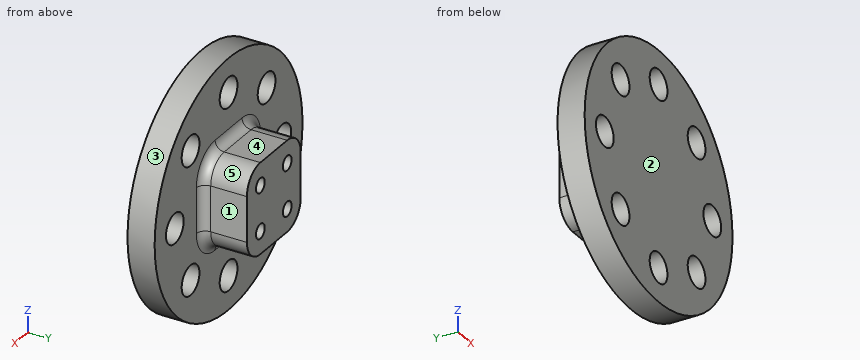
Autodesk Inventor part; units mm, degrees
ref_plane "YZ Plane" through (0, 0, 0) normal (1, 0, 0) x (0, 1, 0)
ref_plane "XZ Plane" through (0, 0, 0) normal (0, 1, 0) x (-1, 0, 0)
ref_plane "XY Plane" through (0, 0, 0) normal (0, 0, 1) x (1, 0, 0)
sketch "Sketch1" plane through (0, 0, 0) normal (0, 1, 0) x (-1, 0, 0)
  circle A0 centre (0, 0) radius 27.5
  dimension "d0" = 55
extrude "Extrusion1" add sketch "Sketch1" along normal blind 6
sketch "Sketch2" plane through (0, 6, 0) normal (0, 1, 0) x (1, 0, 0)
  circle A0 centre (0, 0) radius 27.5
  point P0 (20, 0)
  point P1 (14.1421, 14.1421)
  point P2 (0, 20)
  point P3 (-14.1421, 14.1421)
  point P4 (-20, 0)
  point P5 (-14.1421, -14.1421)
  point P6 (0, -20)
  point P7 (14.1421, -14.1421)
  dimension "d3" = 20
  dimension "d6" = 360
hole "Hole1" at (20, 6, 0) at (14.1421, 6, -14.1421) at (0, 6, -20) at (-14.1421, 6, -14.1421) at (-20, 6, 0) at (-14.1421, 6, 14.1421) at (0, 6, 20) at (14.1421, 6, 14.1421) direction (0, -1, 0) diameter 6.6 depth 8 tip angle 118
sketch "Sketch3" plane through (0, 6, 0) normal (0, 1, 0) x (1, 0, 0)
  circle A0 centre (0, 0) radius 27.5
  line L0 (-5, 10) -> (5, 10)
  line L1 (10, 5) -> (10, -5)
  line L2 (5, -10) -> (-5, -10)
  line L3 (-10, -5) -> (-10, 5)
  arc A1 (-5, 10) -> (-10, 5) centre (-5, 5) ccw
  arc A2 (10, 5) -> (5, 10) centre (5, 5) ccw
  arc A3 (5, -10) -> (10, -5) centre (5, -5) ccw
  arc A4 (-10, -5) -> (-5, -10) centre (-5, -5) ccw
  point P0 (0, 10)
  point P1 (10, 0)
  dimension "d15" = 5
  dimension "d16" = 20
  dimension "d17" = 20
extrude "Extrusion2" add sketch "Sketch3" along normal blind 10 contours L0 A2 L1 A3 L2 A4 L3 A1
sketch "Sketch4" plane through (0, 16, 0) normal (0, 1, 0) x (1, 0, 0)
  arc A0 (-5, 10) -> (-10, 5) centre (-5, 5) ccw
  arc A1 (-10, -5) -> (-5, -10) centre (-5, -5) ccw
  arc A2 (5, -10) -> (10, -5) centre (5, -5) ccw
  arc A3 (10, 5) -> (5, 10) centre (5, 5) ccw
  point P0 (0, 0)
hole "Hole2" at (-5, 16, -5) at (5, 16, -5) at (5, 16, 5) at (-5, 16, 5) direction (0, -1, 0) diameter 3.242 depth 15 tip angle 118
fillet "Fillet1" radius 2 8 edges at (8.5355, 6, -8.5355) (10, 6, 0) (8.5355, 6, 8.5355) (0, 6, 10) (-8.5355, 6, 8.5355) (-10, 6, 0) (-8.5355, 6, -8.5355) (0, 6, -10)
properties part number "simple_holder_right_angle"
Here's how the part is built. I have some questions about the finished solid (model axes, mm). Face numbers are marked on the shaded views. A direction names the side the tool comes from. Coordinates: 2 decimals unless noted, no trailing zeros. Order: outer loops, then holes, each group sorted by start corner. A loop starts at its lowest first (then second) coordinate and runs counter-clockwise, first axis right, second up.
Item 1: If we section it at C-C, the plane z = 20: List the corners of the cut face in (x, y) for me, then the cut area to 3 significant figures.
Response values:
outline: (-18.87, 0) - (-3.3, 0) - (-3.3, 6) - (-18.87, 6) - close; (3.3, 0) - (18.87, 0) - (18.87, 6) - (3.3, 6) - close
area: 187 mm2
Item 2: If we section it at D-D, the plane x = -22: List the corners of the cut face in (y, z) for me, then the cut area to 3 significant figures.
Response values:
outline: (0, -16.5) - (6, -16.5) - (6, -2.62) - (0, -2.62) - close; (0, 2.62) - (6, 2.62) - (6, 16.5) - (0, 16.5) - close
area: 167 mm2
Item 3: If we section it at B-B, the plane y = 15.25: List the corners of the cut face in (x, z) for me, then the cut area to 3 significant figures.
Response values:
outline: (-10, -5) arc R5 ccw to (-5, -10) - (5, -10) arc R5 ccw to (10, -5) - (10, 5) arc R5 ccw to (5, 10) - (-5, 10) arc R5 ccw to (-10, 5) - close; hole circle Ø3.24 at (-5, -5); hole circle Ø3.24 at (-5, 5); hole circle Ø3.24 at (5, -5); hole circle Ø3.24 at (5, 5)
area: 346 mm2
Item 4: I'm going to push flat-ended pins straight in: pin 1 Ø6 at (y, z) = (14, 2) entering from -X; pin 2 Ø4 at (x, z) = (-5, 5) entering from +Y; pin 3 Ø6.5 at (x, y) = (-0.5, 13) entering from -Z; pin 4 Ø6 at (x, y) = (-2, 13) entering from +Z. Where does each tip first touch, or does it pass through?
Response values:
pin 1: stops at x = -10
pin 2: stops at y = 16
pin 3: stops at z = -10
pin 4: stops at z = 10
Item 5: If we section it at A-A, the plane x = 0: List the corners of the cut face in (y, z) for me.
Response values:
outline: (0, -27.5) - (6, -27.5) - (6, -23.3) - (0, -23.3) - close; (0, -16.7) - (6, -16.7) - (6, -12) arc R2 cw to (8, -10) - (16, -10) - (16, 10) - (8, 10) arc R2 cw to (6, 12) - (6, 16.7) - (0, 16.7) - close; (0, 23.3) - (6, 23.3) - (6, 27.5) - (0, 27.5) - close
Item 6: I need wall thicknesses on probe 1 along Z at (x, y) = (0, 5); probe 2 along X at (y, z) = (10.5, 5). Which ranges of each line are inside material? Lowest first, please.
Response values:
probe 1: z = -27.5 to -23.3, -16.7 to 16.7, 23.3 to 27.5
probe 2: x = -10 to -6.62, -3.38 to 3.38, 6.62 to 10
Item 7: Which directions (+Z, -Z, +X, -X, +Y, -Y) give clear straight access to the entire face, cutting with the end or side of a thin tool? Please do the marked faces 1, 2, 3, 4 and 5.
Response values:
face 1: +Z, -Z, +X, +Y
face 2: +Z, -Z, +X, -X, -Y
face 3: +Y, -Y
face 4: +Z, +X, -X, +Y
face 5: +Z, +X, +Y
